The model under review builds one solid part; all positions refer to its coordinate system, in mm. A direction names the side the tool comes from. Give positions to 0.01 mm unless a question says otherwise; leave off trailing zeros. Write each loop counter-clockwise with the first axis right and the second up, starting at its lowest first coordinate (ties: lowest second). Pieces come first, ordered by that corner, then holes.
from build123d import *

# Parameters (mm, degrees)
BOSS_EXTRUDE1_DEPTH     = 3
FILLET4_R               = 8
FILLET5_R               = 3
SKETCH4_R               = 10
BOSS_EXTRUDE4_DEPTH     = 60
CHAMFER2_SIZE           = 17
CHAMFER2_SIZE2          = 42.076476508
FILLET7_R               = 4
FILLET8_R               = 3
SKETCH6_R               = 8.43
CUT_EXTRUDE2_DEPTH      = 15
CUT_EXTRUDE3_DEPTH      = 15
CUT_EXTRUDE3_DEPTH_BACK = 15


with BuildPart() as part:
    # Sketch1 → Boss-Extrude1 (new body)
    with BuildSketch(Plane(origin=(0, 0, 0), x_dir=(1, 0, 0), z_dir=(0, 1, 0))):
        with BuildLine():
            ThreePointArc((29.158991571, 15), (31.870032918, 7.716721534), (32.790955909, 0))
            Line((32.790955909, 0), (95, 0))
            Line((95, 0), (95, 15))
            Line((95, 15), (29.158991571, 15))
        make_face()
        with BuildLine():
            Line((95, 0), (32.790955909, 0))
            ThreePointArc((32.790955909, 0), (31.870032918, -7.716721534), (29.158991571, -15))
            Line((29.158991571, -15), (95, -15))
            Line((95, -15), (95, 0))
        make_face()
        with BuildLine():
            ThreePointArc((15, 29.158991571), (7.716721534, 31.870032918), (0, 32.790955909))
            Line((0, 32.790955909), (0, 0))
            Line((0, 0), (32.790955909, 0))
            ThreePointArc((32.790955909, 0), (31.870032918, 7.716721534), (29.158991571, 15))
            ThreePointArc((29.158991571, 15), (23.186707285, 23.186707285), (15, 29.158991571))
        make_face()
        with BuildLine():
            Line((0, 0), (0, 32.790955909))
            ThreePointArc((0, 32.790955909), (-7.716721534, 31.870032918), (-15, 29.158991571))
            ThreePointArc((-15, 29.158991571), (-23.186707285, 23.186707285), (-29.158991571, 15))
            ThreePointArc((-29.158991571, 15), (-31.870032918, 7.716721534), (-32.790955909, 0))
            Line((-32.790955909, 0), (0, 0))
        make_face()
        with BuildLine():
            Line((32.790955909, 0), (0, 0))
            Line((0, 0), (0, -32.790955909))
            ThreePointArc((0, -32.790955909), (7.716721534, -31.870032918), (15, -29.158991571))
            ThreePointArc((15, -29.158991571), (23.186707285, -23.186707285), (29.158991571, -15))
            ThreePointArc((29.158991571, -15), (31.870032918, -7.716721534), (32.790955909, 0))
        make_face()
        with BuildLine():
            Line((0, -32.790955909), (0, 0))
            Line((0, 0), (-32.790955909, 0))
            ThreePointArc((-32.790955909, 0), (-31.870032918, -7.716721534), (-29.158991571, -15))
            ThreePointArc((-29.158991571, -15), (-23.186707285, -23.186707285), (-15, -29.158991571))
            ThreePointArc((-15, -29.158991571), (-7.716721534, -31.870032918), (0, -32.790955909))
        make_face()
        with BuildLine():
            ThreePointArc((15, 29.158991571), (7.716721534, 31.870032918), (0, 32.790955909))
            Line((0, 32.790955909), (0, 0))
            Line((0, 0), (32.790955909, 0))
            ThreePointArc((32.790955909, 0), (31.870032918, 7.716721534), (29.158991571, 15))
            ThreePointArc((29.158991571, 15), (23.186707285, 23.186707285), (15, 29.158991571))
        make_face()
        with BuildLine():
            Line((0, 0), (0, 32.790955909))
            ThreePointArc((0, 32.790955909), (-7.716721534, 31.870032918), (-15, 29.158991571))
            ThreePointArc((-15, 29.158991571), (-23.186707285, 23.186707285), (-29.158991571, 15))
            ThreePointArc((-29.158991571, 15), (-31.870032918, 7.716721534), (-32.790955909, 0))
            Line((-32.790955909, 0), (0, 0))
        make_face()
        with BuildLine():
            Line((32.790955909, 0), (0, 0))
            Line((0, 0), (0, -32.790955909))
            ThreePointArc((0, -32.790955909), (7.716721534, -31.870032918), (15, -29.158991571))
            ThreePointArc((15, -29.158991571), (23.186707285, -23.186707285), (29.158991571, -15))
            ThreePointArc((29.158991571, -15), (31.870032918, -7.716721534), (32.790955909, 0))
        make_face()
        with BuildLine():
            Line((0, -32.790955909), (0, 0))
            Line((0, 0), (-32.790955909, 0))
            ThreePointArc((-32.790955909, 0), (-31.870032918, -7.716721534), (-29.158991571, -15))
            ThreePointArc((-29.158991571, -15), (-23.186707285, -23.186707285), (-15, -29.158991571))
            ThreePointArc((-15, -29.158991571), (-7.716721534, -31.870032918), (0, -32.790955909))
        make_face()
        with BuildLine():
            ThreePointArc((15, 29.158991571), (7.716721534, 31.870032918), (0, 32.790955909))
            Line((0, 32.790955909), (0, 0))
            Line((0, 0), (32.790955909, 0))
            ThreePointArc((32.790955909, 0), (31.870032918, 7.716721534), (29.158991571, 15))
            ThreePointArc((29.158991571, 15), (23.186707285, 23.186707285), (15, 29.158991571))
        make_face()
        with BuildLine():
            Line((0, 0), (0, 32.790955909))
            ThreePointArc((0, 32.790955909), (-7.716721534, 31.870032918), (-15, 29.158991571))
            ThreePointArc((-15, 29.158991571), (-23.186707285, 23.186707285), (-29.158991571, 15))
            ThreePointArc((-29.158991571, 15), (-31.870032918, 7.716721534), (-32.790955909, 0))
            Line((-32.790955909, 0), (0, 0))
        make_face()
        with BuildLine():
            Line((32.790955909, 0), (0, 0))
            Line((0, 0), (0, -32.790955909))
            ThreePointArc((0, -32.790955909), (7.716721534, -31.870032918), (15, -29.158991571))
            ThreePointArc((15, -29.158991571), (23.186707285, -23.186707285), (29.158991571, -15))
            ThreePointArc((29.158991571, -15), (31.870032918, -7.716721534), (32.790955909, 0))
        make_face()
        with BuildLine():
            Line((0, -32.790955909), (0, 0))
            Line((0, 0), (-32.790955909, 0))
            ThreePointArc((-32.790955909, 0), (-31.870032918, -7.716721534), (-29.158991571, -15))
            ThreePointArc((-29.158991571, -15), (-23.186707285, -23.186707285), (-15, -29.158991571))
            ThreePointArc((-15, -29.158991571), (-7.716721534, -31.870032918), (0, -32.790955909))
        make_face()
        with BuildLine():
            ThreePointArc((15, 29.158991571), (7.716721534, 31.870032918), (0, 32.790955909))
            Line((0, 32.790955909), (0, 0))
            Line((0, 0), (32.790955909, 0))
            ThreePointArc((32.790955909, 0), (31.870032918, 7.716721534), (29.158991571, 15))
            ThreePointArc((29.158991571, 15), (23.186707285, 23.186707285), (15, 29.158991571))
        make_face()
        with BuildLine():
            Line((0, 0), (0, 32.790955909))
            ThreePointArc((0, 32.790955909), (-7.716721534, 31.870032918), (-15, 29.158991571))
            ThreePointArc((-15, 29.158991571), (-23.186707285, 23.186707285), (-29.158991571, 15))
            ThreePointArc((-29.158991571, 15), (-31.870032918, 7.716721534), (-32.790955909, 0))
            Line((-32.790955909, 0), (0, 0))
        make_face()
        with BuildLine():
            Line((32.790955909, 0), (0, 0))
            Line((0, 0), (0, -32.790955909))
            ThreePointArc((0, -32.790955909), (7.716721534, -31.870032918), (15, -29.158991571))
            ThreePointArc((15, -29.158991571), (23.186707285, -23.186707285), (29.158991571, -15))
            ThreePointArc((29.158991571, -15), (31.870032918, -7.716721534), (32.790955909, 0))
        make_face()
        with BuildLine():
            Line((0, -32.790955909), (0, 0))
            Line((0, 0), (-32.790955909, 0))
            ThreePointArc((-32.790955909, 0), (-31.870032918, -7.716721534), (-29.158991571, -15))
            ThreePointArc((-29.158991571, -15), (-23.186707285, -23.186707285), (-15, -29.158991571))
            ThreePointArc((-15, -29.158991571), (-7.716721534, -31.870032918), (0, -32.790955909))
        make_face()
        with BuildLine():
            Line((0, 32.790955909), (0, 95))
            Line((0, 95), (-15, 95))
            Line((-15, 95), (-15, 29.158991571))
            ThreePointArc((-15, 29.158991571), (-7.716721534, 31.870032918), (0, 32.790955909))
        make_face()
        with BuildLine():
            Line((15, 95), (0, 95))
            Line((0, 95), (0, 32.790955909))
            ThreePointArc((0, 32.790955909), (7.716721534, 31.870032918), (15, 29.158991571))
            Line((15, 29.158991571), (15, 95))
        make_face()
        with BuildLine():
            Line((-95, 0), (-32.790955909, 0))
            ThreePointArc((-32.790955909, 0), (-31.870032918, 7.716721534), (-29.158991571, 15))
            Line((-29.158991571, 15), (-95, 15))
            Line((-95, 15), (-95, 0))
        make_face()
        with BuildLine():
            ThreePointArc((-29.158991571, -15), (-31.870032918, -7.716721534), (-32.790955909, 0))
            Line((-32.790955909, 0), (-95, 0))
            Line((-95, 0), (-95, -15))
            Line((-95, -15), (-29.158991571, -15))
        make_face()
        with BuildLine():
            Line((0, -95), (0, -32.790955909))
            ThreePointArc((0, -32.790955909), (-7.716721534, -31.870032918), (-15, -29.158991571))
            Line((-15, -29.158991571), (-15, -95))
            Line((-15, -95), (0, -95))
        make_face()
        with BuildLine():
            ThreePointArc((15, -29.158991571), (7.716721534, -31.870032918), (0, -32.790955909))
            Line((0, -32.790955909), (0, -95))
            Line((0, -95), (15, -95))
            Line((15, -95), (15, -29.158991571))
        make_face()
    extrude(amount=BOSS_EXTRUDE1_DEPTH)

    # Fillet4
    fillet4_edges = [part.edges().sort_by_distance(p)[0] for p in [
        (95, 1.5, -15),
        (95, 1.5, 15),
        (15, 1.5, 95),
        (-15, 1.5, 95),
        (-95, 1.5, 15),
        (-95, 1.5, -15),
        (-15, 1.5, -95),
        (15, 1.5, -95),
    ]]
    fillet(fillet4_edges, radius=FILLET4_R)

    # Fillet5
    fillet5_edges = [part.edges().sort_by_distance(p)[0] for p in [
        (-12.656854249, 3, 92.656854249),
        (-15, 3, 58.079495785),
        (-23.186707285, 3, 23.186707285),
        (-58.079495785, 3, 15),
        (-92.656854249, 3, 12.656854249),
        (-95, 3, 0),
        (-92.656854249, 3, -12.656854249),
        (-58.079495785, 3, -15),
        (-23.186707285, 3, -23.186707285),
        (-15, 3, -58.079495785),
        (-12.656854249, 3, -92.656854249),
        (0, 3, -95),
        (12.656854249, 3, -92.656854249),
        (15, 3, -58.079495785),
        (23.186707285, 3, -23.186707285),
        (58.079495785, 3, -15),
        (92.656854249, 3, -12.656854249),
        (95, 3, 0),
        (92.656854249, 3, 12.656854249),
        (58.079495785, 3, 15),
        (23.186707285, 3, 23.186707285),
        (15, 3, 58.079495785),
        (12.656854249, 3, 92.656854249),
        (0, 3, 95),
    ]]
    fillet(fillet5_edges, radius=FILLET5_R - 0.0001)  # a hair under: the kernel refuses the full size

    # Sketch4 → Boss-Extrude4 (add)
    with BuildSketch(Plane(origin=(0, 3, 0), x_dir=(1, 0, 0), z_dir=(0, 1, 0))):
        with Locations(Location((0, 0, 0), (0, 0, 270))):
            Circle(SKETCH4_R)
    extrude(amount=BOSS_EXTRUDE4_DEPTH)

    # Chamfer2
    chamfer2_edges = [part.edges().sort_by_distance(p)[0] for p in [
        (0, 3, -10),
    ]]
    chamfer2_side = [part.faces().sort_by_distance(p)[0] for p in [
        (9.397944217, 3, 57.133640491),
    ]]
    chamfer(chamfer2_edges, length=CHAMFER2_SIZE, length2=CHAMFER2_SIZE2, reference=chamfer2_side[0])

    # Fillet7
    fillet7_edges = [part.edges().sort_by_distance(p)[0] for p in [
        (0, 45.076476508, -10),
    ]]
    fillet(fillet7_edges, radius=FILLET7_R)

    # Fillet8
    fillet8_edges = [part.edges().sort_by_distance(p)[0] for p in [
        (0, 3, -27),
    ]]
    fillet(fillet8_edges, radius=FILLET8_R)

    # Sketch6 → Cut-Extrude2 (cut)
    with BuildSketch(Plane(origin=(0, 63, 0), x_dir=(1, 0, 0), z_dir=(0, 1, 0))):
        with Locations(Location((0, 0, 0), (0, 0, 270))):
            Circle(SKETCH6_R)
    extrude(amount=-CUT_EXTRUDE2_DEPTH, mode=Mode.SUBTRACT)

    # Sketch8 → Cut-Extrude3 (cut, two sides: drawn at the far end of the back side and taken through both)
    with BuildSketch(Plane(origin=(0, 0, 0), x_dir=(0, 0, -1), z_dir=(1, 0, 0)).offset(-CUT_EXTRUDE3_DEPTH_BACK)):
        with BuildLine():
            Line((0, 55.5), (0, 57.1))
            ThreePointArc((0, 57.1), (-1.6, 55.5), (0, 53.9))
            Line((0, 53.9), (0, 55.5))
        make_face()
        with BuildLine():
            ThreePointArc((1.6, 55.5), (1.13137085, 56.63137085), (0, 57.1))
            Line((0, 57.1), (0, 55.5))
            Line((0, 55.5), (1.6, 55.5))
        make_face()
        with BuildLine():
            Line((1.6, 55.5), (0, 55.5))
            Line((0, 55.5), (0, 53.9))
            ThreePointArc((0, 53.9), (1.13137085, 54.36862915), (1.6, 55.5))
        make_face()
        with BuildLine():
            ThreePointArc((1.6, 55.5), (1.13137085, 56.63137085), (0, 57.1))
            Line((0, 57.1), (0, 55.5))
            Line((0, 55.5), (1.6, 55.5))
        make_face()
        with BuildLine():
            Line((1.6, 55.5), (0, 55.5))
            Line((0, 55.5), (0, 53.9))
            ThreePointArc((0, 53.9), (1.13137085, 54.36862915), (1.6, 55.5))
        make_face()
    extrude(amount=CUT_EXTRUDE3_DEPTH + CUT_EXTRUDE3_DEPTH_BACK, mode=Mode.SUBTRACT)


solid = part.part
1) Insertion check: pin 1 (4 mm diameter, centred on y = 11, z = -19, fed in from +X); pin 2 (13.5 mm diameter, centred on x = 0, z = 0, fed in from +Y); pin 3 (10 mm diameter, centred on x = 1, y = 18, fed in from -Z). Each pin has a flat end and moves straight along its axis. Give the tip position at first contact, or say it passes through.
2) The part is to be moulded in two halves that separate along Z. For faces 3 (the flat face through (0, 48, 0)), 4 (the flat face through (-20.9, 3, -20.9)), 5 (the conical face through (-9.97, 29.28, -13)), say which applies: +Z half, -Z half, draft (parallel to the pull), parting line (faces both ways), or undercut.
3) Consider section D-D, the plane y = 25. Give the boundary of the cut face in (x, z).
4) Tool access review of faces 1 (the flat face through (-7, 63, -5)), 2 (the cylindrical face through (-8.23, 55.6, -1.83)): name each direction out of +Z, -Z, +X, -X, +Y, -Y from which nothing blocks a thin tool from reaching the whole face with its end or side.
5) To check wall thickness, follow probe 1 along Y at (x, z) = (65, -10); probe 2 along Z at (x, y) = (-2, 55); probe 3 along X at (y, z) = (19, 16). State the ranges of each line that lie inside material, in increasing order.
6) Consider section A-A, the plane y = 51. Give the boundary of the cut face in (x, z).
Answer block:
1. pin 1: stops at x = 16.91
1. pin 2: stops at y = 48
1. pin 3: stops at z = -22.95
2. face 3: undercut
2. face 4: draft
2. face 5: parting line
3. outline: circle Ø36.22 at (0, 0)
4. face 1: +Z, -Z, +X, -X, +Y
4. face 2: +Y
5. probe 1: y = 0 to 3
5. probe 2: z = -9.8 to -8.19, 8.19 to 9.8
5. probe 3: x = -12.87 to 12.87
6. outline: circle Ø20 at (0, 0); hole circle Ø16.86 at (0, 0)
